Could you check a few things on this model? Use its own coordinates, in mm. Face numbers are marked on the shaded views. A direction names the side the tool comes from. Round coordinates to 2 decimals unless told otherwise and drop trailing zeros. Loops run counter-clockwise (first coordinate to the right, second up) from the corner with the lowest first, then second, coordinate; pieces in that order, holes last.
from build123d import *

# Parameters (mm, degrees)
F2_R    = 0.0508
F3_SIZE = 0.127


with BuildPart() as f1:
    # F0 (on Right) → F1 (revolve)
    with BuildSketch(Plane.YZ):
        Polygon((-3.175, -2.54), (0, -2.54), (0, 0), (0, 5.206), (-3.175, 5.206), (-3.175, 8), (-19.05, 8), (-19.05, 0), (-3.175, 0), align=None)
    revolve(axis=Axis((0, 0, 2.603), (0, 0, -1)))

    # F2
    f2_edges = [f1.edges().sort_by_distance(p)[0] for p in [
        (0, 3.175, 0),
    ]]
    fillet(f2_edges, radius=F2_R)

    # F3
    f3_edges = [f1.edges().sort_by_distance(p)[0] for p in [
        (0, 19.05, 0),
        (0, 19.05, 8),
        (0, 3.175, 8),
    ]]
    chamfer(f3_edges, length=F3_SIZE)


solid = f1.part
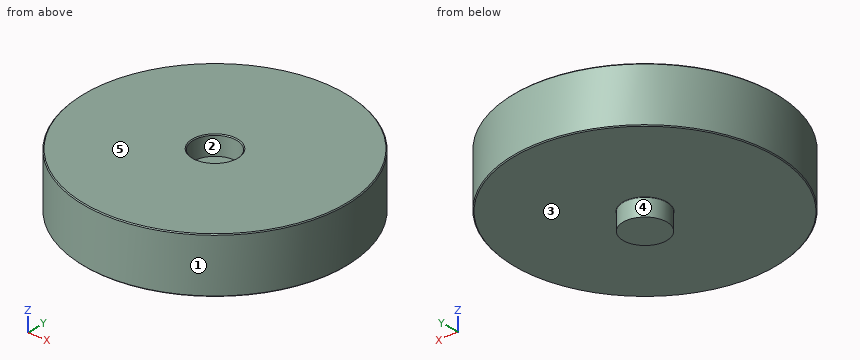
Item 1: We'd pull the mould along X, two halves only. Please class the marked faces 1, 2 and 3: released by +X, released by -X, zero draft, split by the parting line, or undercut.
Results list:
face 1: split by the parting line
face 2: undercut
face 3: zero draft
Item 2: If we section it at C-C, the plane z = 3.5: Please give me the cut outline in (x, y).
Results list:
outline: circle Ø38.1 at (0, 0)
Item 3: If I drill on line 1 along Y through (x, z) = (0, 6) (3 decimals); line 2 along Z through (x, y) = (-10, -5.5), over which ranges is the centre line in solid material (lowest first)?
Results list:
line 1: y = -19.05 to -3.175, 3.175 to 19.05
line 2: z = 0 to 8
Item 4: Will these pins go through, and if not, where does the flat tip stop? pin 1 (3 mm diameter, centred on x = -1, y = -1, fed in from +Z); pin 2 (4 mm diameter, centred on y = 7.5, z = 3, fed in from +X); pin 3 (5 mm diameter, centred on x = 9.5, z = 4.5, fed in from -Y).
Results list:
pin 1: stops at z = 5.21
pin 2: stops at x = 18.24
pin 3: stops at y = -17.72
Item 5: If we section it at A-A, the plane y = 0: Please give me the cut outline in (x, z) (3 decimals), then the cut area to 3 significant figures.
Results list:
outline: (-19.05, 0.127) - (-18.923, 0) - (-3.226, 0) arc R0.051 cw to (-3.175, -0.051) - (-3.175, -2.54) - (3.175, -2.54) - (3.175, -0.051) arc R0.051 cw to (3.226, 0) - (18.923, 0) - (19.05, 0.127) - (19.05, 7.873) - (18.923, 8) - (3.302, 8) - (3.175, 7.873) - (3.175, 5.206) - (-3.175, 5.206) - (-3.175, 7.873) - (-3.302, 8) - (-18.923, 8) - (-19.05, 7.873) - close
area: 303 mm2
Item 6: For the marked faces 4 and 5, which set-ups out of +Z, -Z, +X, -X, +Y, -Y let a thin tool reach every point of the face, with its end or its side?
Results list:
face 4: -Z
face 5: +Z, +X, -X, +Y, -Y
